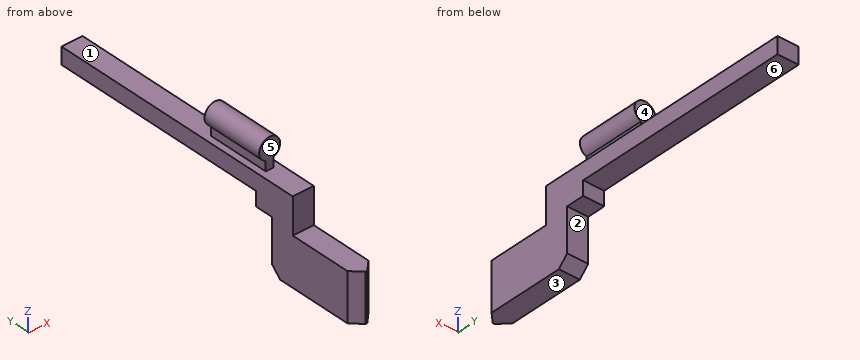
```python
from build123d import *

# Parameters (mm, degrees)
SZKIC1_W                    = 4.4
SZKIC1_H                    = 21
DODANIE_WYCI_GNI_CIE1_DEPTH = 6.5
SZKIC3_R                    = 2.2
SZKIC3_W                    = 1.65
SZKIC3_H                    = 4.05
DODANIE_WYCI_GNI_CIE2_DEPTH = 13
SKETCH1_W                   = 4.4
SKETCH1_H                   = 5
BOSS_EXTRUDE1_DEPTH         = 11
SKETCH3_W                   = 4.4
SKETCH3_H                   = 10
BOSS_EXTRUDE3_DEPTH         = 15
CHAMFER1_SIZE               = 2
SKETCH5_W                   = 4.4
SKETCH5_H                   = 3
CUT_EXTRUDE1_DEPTH          = 12.2
SZKIC4_W                    = 4.4
SZKIC4_H                    = 3.5
DODANIE_WYCI_GNI_CIE3_DEPTH = 34


with BuildPart() as part:
    # Szkic1 → Dodanie-wyciągnięcie1 (new body)
    with BuildSketch(Plane.XY):
        Rectangle(SZKIC1_W, SZKIC1_H)
    extrude(amount=DODANIE_WYCI_GNI_CIE1_DEPTH)

    # Szkic3 → Dodanie-wyciągnięcie2 (add)
    with BuildSketch(Plane(origin=(0, 10.5, 0), x_dir=(1, 0, 0), z_dir=(0, 1, 0))):
        with Locations((0, -10.55)):
            Circle(SZKIC3_R)
        with Locations((0, -8.525)):
            Rectangle(SZKIC3_W, SZKIC3_H)
    extrude(amount=-DODANIE_WYCI_GNI_CIE2_DEPTH)

    # Sketch1 → Boss-Extrude1 (add)
    with BuildSketch(Plane(origin=(0, 0, 0), x_dir=(-1, 0, 0), z_dir=(0, 0, -1))):
        with Locations((0, -8)):
            Rectangle(SKETCH1_W, SKETCH1_H)
    extrude(amount=BOSS_EXTRUDE1_DEPTH)

    # Sketch3 → Boss-Extrude3 (add)
    with BuildSketch(Plane.XZ.offset(10.5)):
        with Locations((0, -6)):
            Rectangle(SKETCH3_W, SKETCH3_H)
    extrude(amount=BOSS_EXTRUDE3_DEPTH)

    # Chamfer1
    chamfer1_edges = [part.edges().sort_by_distance(p)[0] for p in [
        (0, -5.5, -11),
        (2.2, -25.5, -6),
        (-2.2, -25.5, -6),
    ]]
    chamfer(chamfer1_edges, length=CHAMFER1_SIZE)

    # Sketch5 → Cut-Extrude1 (cut)
    with BuildSketch(Plane(origin=(0, 10.5, 0), x_dir=(1, 0, 0), z_dir=(0, 1, 0))):
        with Locations((0, -1.5)):
            Rectangle(SKETCH5_W, SKETCH5_H)
    extrude(amount=-CUT_EXTRUDE1_DEPTH, mode=Mode.SUBTRACT)

    # Szkic4 → Dodanie-wyciągnięcie3 (add)
    with BuildSketch(Plane(origin=(0, 10.5, 0), x_dir=(1, 0, 0), z_dir=(0, 1, 0))):
        with Locations((0, -4.75)):
            Rectangle(SZKIC4_W, SZKIC4_H)
    extrude(amount=DODANIE_WYCI_GNI_CIE3_DEPTH)


solid = part.part
```
Verification items for the finished model (mm, model axes). Face numbers are marked on the shaded views. A direction names the side the tool comes from. Coordinates: 2 decimals unless noted, no trailing zeros. Write each loop counter-clockwise with the first axis right and the second up, starting at its lowest first coordinate (ties: lowest second). Pieces come first, ordered by that corner, then holes. Notation, with made-up numbers: M 85.25,-23 L 138.25,-23 A31 cw 138.25,4 Z; hole C -5,-34.5 d8. An arc over 180 degrees is marked long. Answer as a JSON object with one key per item and string values. Group by question number.
(1) Cross-section at A-A, the plane y = 3. Record the cut outline in (x, z) (3 decimals).
(2) Material ranges on line 1 (Z direction, x = -1.1, y = -12); line 2 (Z direction, x = 0.25, y = 21); line 3 (Y direction, x = -0.5, z = 1.5), recorded low to high.
(3) Release check for a two-part mould opening along Z. For the marked faces 1, 2 and 3 record: +Z half, -Z half, draft (parallel to the pull), parting line (faces both ways), or undercut.
(4) Tool access check on the marked faces 4, 5 and 6. Record the directions out of +Z, -Z, +X, -X, +Y, -Y that give a thin tool (end or side, any length) a straight path to the whole face; none if there is none.
(5) Gauge pin test, flat ends, axial feed: pin 1 (1.5 mm diameter, centred on x = 0, y = 36, fed in from -Z); pin 2 (1.3 mm diameter, centred on x = 0, z = 9, fed in from -Y); pin 3 (1.5 mm diameter, centred on x = 0.5, z = 1, fed in from +Y); pin 4 (2 mm diameter, centred on y = 3.5, z = 7, fed in from +X). Record the tip position at first contact, or that the pin passes through.
(6) Cross-section at B-B, the plane z = -4. Record the cut outline in (x, y).
(7) Cross-section at C-C, the plane z = 10.55. Record the cut outline in (x, y), and give its area (3 significant figures).
Reply:
{
 "1": {"outline": "M -2.2,3 L 2.2,3 L 2.2,6.5 L 0.825,6.5 L 0.825,8.511 A2.2 ccw long -0.825,8.511 L -0.825,6.5 L -2.2,6.5 Z"},
 "2": {"line 1": "-11 to -1", "line 2": "3 to 6.5", "line 3": "-10.5 to -1.7"},
 "3": {"face 1": "undercut", "face 2": "draft", "face 3": "-Z half"},
 "4": {"face 4": "+Z, +X, -X, +Y", "face 5": "+Z, +X, -X, -Y", "face 6": "-Z, +X, -X, +Y"},
 "5": {"pin 1": "z = 3", "pin 2": "y = -2.5", "pin 3": "y = -1.7", "pin 4": "x = 2.2"},
 "6": {"outline": "M -2.2,-23.5 L -0.2,-25.5 L 0.2,-25.5 L 2.2,-23.5 L 2.2,-5.5 L -2.2,-5.5 Z"},
 "7": {"outline": "M -2.2,-2.5 L 2.2,-2.5 L 2.2,10.5 L -2.2,10.5 Z", "area": "57.2 mm²"}
}
